from build123d import *

# Parameters (mm, degrees)
SKETCH1_R           = 1.2
BOSS_EXTRUDE1_DEPTH = 4.8
SKETCH2_R           = 2
CUT_EXTRUDE1_DEPTH  = 1.8
FILLET1_R           = 1


with BuildPart() as part:
    # Sketch1 → Boss-Extrude1 (new body)
    with BuildSketch(Plane.XY):
        with BuildLine():
            Line((5, -2), (55, -2))
            ThreePointArc((55, -2), (56.961161351, -2.194193243), (58.846153846, -2.769230769))
            ThreePointArc((58.846153846, -2.769230769), (63, 0), (58.846153846, 2.769230769))
            ThreePointArc((58.846153846, 2.769230769), (56.961161351, 2.194193243), (55, 2))
            Line((55, 2), (5, 2))
            ThreePointArc((5, 2), (3.038838649, 2.194193243), (1.153846154, 2.769230769))
            ThreePointArc((1.153846154, 2.769230769), (-3, 0), (1.153846154, -2.769230769))
            ThreePointArc((1.153846154, -2.769230769), (3.038838649, -2.194193243), (5, -2))
        make_face()
        Circle(SKETCH1_R, mode=Mode.SUBTRACT)
        with Locations((60, 0)):
            Circle(SKETCH1_R, mode=Mode.SUBTRACT)
    extrude(amount=BOSS_EXTRUDE1_DEPTH)

    # Sketch2 → Cut-Extrude1 (cut)
    with BuildSketch(Plane.XY.offset(4.8)):
        with Locations((60, 0)):
            Circle(SKETCH2_R)
    extrude(amount=-CUT_EXTRUDE1_DEPTH, mode=Mode.SUBTRACT)

    # Fillet1
    # the kernel refuses this fillet: 1 mm, written as the material it adds along each edge
    with BuildSketch(Plane(origin=(60, 0, 3), x_dir=(1, 0, 0), z_dir=(0, -1, 0))) as fillet1_piece_1:
        with BuildLine():
            CenterArc((1, 0.979795897), FILLET1_R, 281.536959033, 78.463040967)
            Line((1.2, 0), (1.204, -0.019595918))
            ThreePointArc((1.204, -0.019595918), (1.6, -0.02), (2, -0.02))
            Line((2, -0.02), (2.02, 0))
            Line((2.02, 0), (2.02, 0.979795897))
            Line((2.02, 0.979795897), (2, 0.979795897))
        make_face()
    revolve(axis=Axis((60, 0, 3), (0, 0, 1)))


solid = part.part
Here's how the part is built. I have some questions about the finished solid (model axes, mm). A direction names the side the tool comes from. Coordinates: 2 decimals unless noted, no trailing zeros. Order: outer loops, then holes, each group sorted by start corner. A loop starts at its lowest first (then second) coordinate and runs counter-clockwise, first axis right, second up. Notation, with made-up numbers: M 35.5,58 L 64.5,58 A20 ccw 64.5,96 Z; hole C 88.25,5 d7. An arc over 180 degrees is marked long. Answer as CSV lines item,"result". Start each with the question number.
1. I need wall thicknesses on line 1 (X direction, y = -0.1, z = 2); line 2 (X direction, y = 0.6, z = 2.15); line 3 (Y direction, x = 60, z = 0.65). Which ranges of each line are inside material? Lowest first, please. Write a range as [from, to].
2. I want a section at A-A, the plane x = 0. Write out the boundary of the cut face in (y, z), and give its area (3 significant figures).
3. We'd pull the mould along Y, two halves only. Please class faces 1 (the cylindrical face through (0.65, 1.01, 2.37)), 2 (the cylindrical face through (56.93, -2.19, 2.37)), 3 (the flat face through (30, 0, 4.8)): released by +Y, released by -Y, zero draft, split by the parting line, or undercut.
4. On a 3-axis mill with a long thin cutter (end or side, diameter ignored), from which of +Z, -Z, +X, -X, +Y, -Y can I reach the whole of each face in a straight line? I mean faces 4 (the cylindrical face through (58.002, 0.088, 4.396)), 5 (the flat face through (30, 2, 2)), 6 (the cylindrical face through (3, -2.2, 2.4)), 7 (the flat face through (30, 0, 0)). Say none if no direction works.
5. For pin 1 (2.5 mm diameter, centred on x = 24, z = 1.5, fed in from -Y); pin 2 (1 mm diameter, centred on x = 45.5, z = 2.5, fed in from +Y), each with a flat end and sliding along its axis, tell me the tip position at first contact or that it passes through.
6. I want a section at C-C, the plane y = 0. Count the separate pieces of the cut face and the enclosed holes in it, and give its area (3 significant figures).
7. I want a section at B-B, the plane z = 1.3. Write out the boundary of the cut face in (x, y).
Recorded:
1,line 1,"x = [-3, -1.2], [1.2, 58.8], [61.2, 63]"
1,line 2,"x = [-2.94, -1.04], [1.04, 58.96], [61.04, 62.94]"
1,line 3,"y = [-3, -1.2], [1.2, 3]"
2,outline,"M -3,0 L -1.2,0 L -1.2,4.8 L -3,4.8 Z; M 1.2,0 L 3,0 L 3,4.8 L 1.2,4.8 Z"
2,area,"17.3 mm2"
3,face 1,"undercut"
3,face 2,"released by -Y"
3,face 3,"zero draft"
4,face 4,"+Z"
4,face 5,"+Z, -Z, +Y"
4,face 6,"+Z, -Z, -Y"
4,face 7,"-Z, +X, -X, +Y, -Y"
5,pin 1,"stops at y = -2"
5,pin 2,"stops at y = 2"
6,separate pieces,"3"
6,enclosed holes,"0"
6,area,"291 mm2"
7,outline,"M 1.15,-2.77 A10 cw 5,-2 L 55,-2 A10 cw 58.85,-2.77 A3 ccw long 58.85,2.77 A10 cw 55,2 L 5,2 A10 cw 1.15,2.77 A3 ccw long Z; hole C 0,0 d2.4; hole C 60,0 d2.4"
